Read the model definition and answer for the solid it produces. Units are mm, in the model's axes. Coordinates: 2 decimals unless noted, no trailing zeros. Order: outer loops, then holes, each group sorted by start corner. A loop starts at its lowest first (then second) coordinate and runs counter-clockwise, first axis right, second up. Notation, with made-up numbers: (-39, 24.25) -> (2, 24.25) arc R10 ccw to (2, 37.25) -> close; hole circle Ø2 at (39.25, 51). An arc over 180 degrees is marked (long way). Answer as a JSON object with one key per item and string values. Group by question number.
1) Section C-C on y = 84.75 is taken. Determine the outline of the cut face in (x, z), and give its area (3 significant figures).
2) Section A-A on y = 92.5 is taken. Determine the outline of the cut face in (x, z), and give its area (3 significant figures).
3) Given pin 1 (1.5 mm diameter, centred on x = 2.5, z = 55, fed in from -Y); pin 2 (2.5 mm diameter, centred on x = 2, z = 36, fed in from +Y); pin 3 (1.5 mm diameter, centred on x = 3, z = 94.5, fed in from -Y), each flat-ended and moving along its own axis, determine where each tip first touches the part or whether it passes through.
4) Section D-D on y = 96.5 is taken. Determine the outline of the cut face in (x, z), and give its area (3 significant figures).
5) Consider L1, parallel to Z at x = 4.4, y = 90.75; L2, parallel to Z at x = 3.1, y = 95.75; L3, parallel to Z at x = 0.75, y = 87.75. Determine where each line is inside the solid, lowest interval first.
from build123d import *

# Parameters (mm, degrees)
BOSS_EXTRUDE1_DEPTH = 5


with BuildPart() as part:
    # Sketch1 → Boss-Extrude1 (new body)
    with BuildSketch(Plane(origin=(0, 0, 0), x_dir=(0, -1, 0), z_dir=(1, 0, 0))):
        with BuildLine():
            Line((-81, -13.4), (-87, -13.4))
            Line((-87, -13.4), (-97.4, -13.4))
            Line((-97.4, -13.4), (-97.4, -2.6))
            Line((-97.4, -2.6), (-87, -2.6))
            Line((-87, -2.6), (-87, -2))
            ThreePointArc((-87, -2), (-87.585786438, -0.585786438), (-89, 0))
            Line((-89, 0), (-98, 0))
            ThreePointArc((-98, 0), (-99.414213562, -0.585786438), (-100, -2))
            Line((-100, -2), (-100, -14))
            ThreePointArc((-100, -14), (-99.414213562, -15.414213562), (-98, -16))
            Line((-98, -16), (-97.5, -16))
            ThreePointArc((-97.5, -16), (-94.671572875, -17.171572875), (-93.5, -20))
            Line((-93.5, -20), (-93.5, -80))
            ThreePointArc((-93.5, -80), (-94.671572875, -82.828427125), (-97.5, -84))
            Line((-97.5, -84), (-98, -84))
            ThreePointArc((-98, -84), (-99.414213562, -84.585786438), (-100, -86))
            Line((-100, -86), (-100, -98))
            ThreePointArc((-100, -98), (-99.414213562, -99.414213562), (-98, -100))
            Line((-98, -100), (-89, -100))
            ThreePointArc((-89, -100), (-87.585786438, -99.414213562), (-87, -98))
            Line((-87, -98), (-87, -97.4))
            Line((-87, -97.4), (-97.4, -97.4))
            Line((-97.4, -97.4), (-97.4, -86.6))
            Line((-97.4, -86.6), (-87, -86.6))
            Line((-87, -86.6), (-81, -86.6))
            Line((-81, -86.6), (-81, -86))
            Line((-81, -86), (-81, -85.99))
            ThreePointArc((-81, -85.99), (-81.582857505, -84.582857505), (-82.99, -84))
            Line((-82.99, -84), (-83, -84))
            Line((-83, -84), (-83.01, -84))
            ThreePointArc((-83.01, -84), (-85.831356057, -82.831356057), (-87, -80.01))
            Line((-87, -80.01), (-87, -80))
            Line((-87, -80), (-87, -20))
            Line((-87, -20), (-87, -19.99))
            ThreePointArc((-87, -19.99), (-85.831356057, -17.168643943), (-83.01, -16))
            Line((-83.01, -16), (-83, -16))
            Line((-83, -16), (-82.99, -16))
            ThreePointArc((-82.99, -16), (-81.582857505, -15.417142495), (-81, -14.01))
            Line((-81, -14.01), (-81, -14))
            Line((-81, -14), (-81, -13.4))
        make_face()
    extrude(amount=BOSS_EXTRUDE1_DEPTH)


solid = part.part
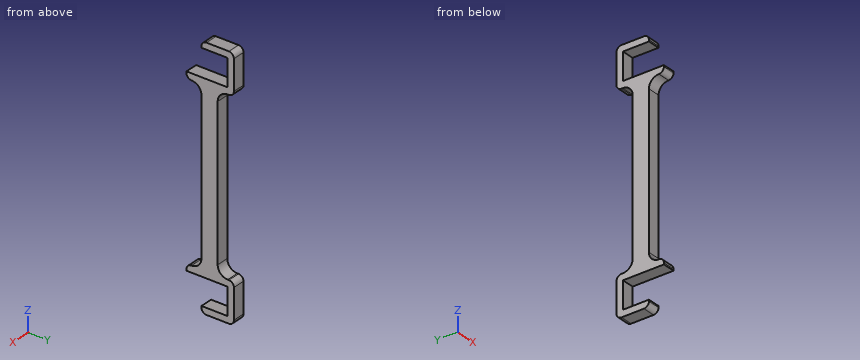
Worked answers:
{
 "1": {"outline": "(0, 13.4) -> (5, 13.4) -> (5, 16.4) -> (0, 16.4) -> close; (0, 83.6) -> (5, 83.6) -> (5, 86.6) -> (0, 86.6) -> close", "area": "30.0 mm²"},
 "2": {"outline": "(0, 0) -> (5, 0) -> (5, 2.6) -> (0, 2.6) -> close; (0, 13.4) -> (5, 13.4) -> (5, 86.6) -> (0, 86.6) -> close; (0, 97.4) -> (5, 97.4) -> (5, 100) -> (0, 100) -> close", "area": "392 mm²"},
 "3": {"pin 1": "stops at y = 87", "pin 2": "stops at y = 93.5", "pin 3": "stops at y = 97.4"},
 "4": {"outline": "(0, 0) -> (5, 0) -> (5, 2.6) -> (0, 2.6) -> close; (0, 13.4) -> (5, 13.4) -> (5, 16.13) -> (0, 16.13) -> close; (0, 83.87) -> (5, 83.87) -> (5, 86.6) -> (0, 86.6) -> close; (0, 97.4) -> (5, 97.4) -> (5, 100) -> (0, 100) -> close", "area": "53.3 mm²"},
 "5": {"L1": "z = 0 to 2.6, 13.4 to 86.6, 97.4 to 100", "L2": "z = 0 to 2.6, 13.4 to 16.4, 83.6 to 86.6, 97.4 to 100", "L3": "z = 0.44 to 2.6, 13.4 to 86.6, 97.4 to 99.56"}
}
